```python
from build123d import *

# Parameters (mm, degrees)
SKETCH1_W           = 28
SKETCH1_H           = 12
BOSS_EXTRUDE1_DEPTH = 5
SKETCH2_W           = 28
SKETCH2_H           = 6
BOSS_EXTRUDE2_DEPTH = 13.5
SKETCH3_R           = 1.75
CUT_EXTRUDE1_DEPTH  = 21.353132437


with BuildPart() as part:
    # Sketch1 → Boss-Extrude1 (new body)
    with BuildSketch(Plane.XY):
        Rectangle(SKETCH1_W, SKETCH1_H)
    extrude(amount=BOSS_EXTRUDE1_DEPTH)

    # Sketch2 → Boss-Extrude2 (add)
    with BuildSketch(Plane.XY.offset(5)):
        with Locations((0, -3)):
            Rectangle(SKETCH2_W, SKETCH2_H)
    extrude(amount=BOSS_EXTRUDE2_DEPTH)

    # Sketch3 → Cut-Extrude1 (cut, through all)
    with BuildSketch(Plane.XY.offset(5)):
        with Locations((-11, 3)):
            Circle(SKETCH3_R)
        with Locations(Location((11, 3, 0), (0, 0, 180))):
            Circle(SKETCH3_R)
    extrude(amount=-CUT_EXTRUDE1_DEPTH, mode=Mode.SUBTRACT)


solid = part.part
```
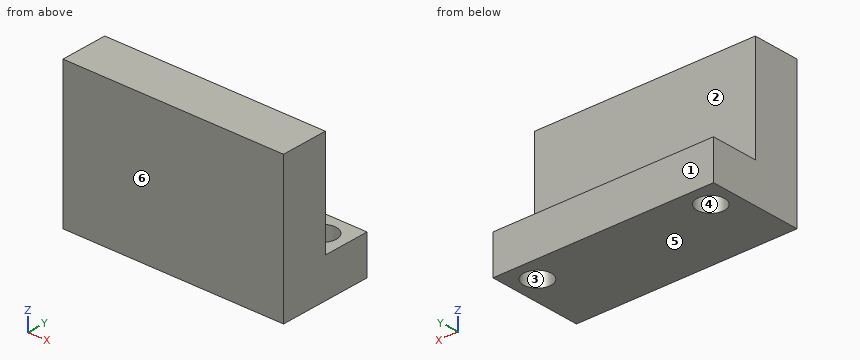
Check sheet for the modelled part. Datum: model origin and axes. Units: mm. Face numbers are marked on the shaded views. A direction names the side the tool comes from. Give positions to 0.01 mm unless a question says otherwise; leave off trailing zeros. Order: outer loops, then holes, each group sorted by start corner. A loop starts at its lowest first (then second) coordinate and runs counter-clockwise, first axis right, second up. Notation, with made-up numbers: M 30.25,18 L 89.25,18 A17 ccw 89.25,34 Z; hole C 71,19.5 d11. An arc over 180 degrees is marked long. Answer in a Markdown table with one row per item. Add a question column.
Q1. Sectioned sample at A-A, the plane x = 11. Record the boundary of the cut face in (y, z), and give its area (4 significant figures).
Q2. Release check for a two-part mould opening along Y. For the marked faces 3, 4, 5 and 6 record: released by +Y, released by -Y, zero draft, split by the parting line, or undercut.
Q3. Thickness scan on L1, parallel to Y at x = -11, z = 3.85; L2, parallel to Z at x = 0.5, y = 0.5; L3, parallel to Y at x = 3.5, z = 13.25. Record the ranges inside material, lowest first.
Q4. Sectioned sample at D-D, the plane x = -4. Record the boundary of the cut face in (y, z).
Q5. Sectioned sample at C-C, the plane z = 2. Record the boundary of the cut face in (x, y), and give its area (3 significant figures).
Q6. Access from +Z, -Z, +X, -X, +Y, -Y to the whole of each face (thin tool, end or side, straight path). Record for the marked faces 1 and 2.
Q7. Gauge pin test, flat ends, axial feed: pin 1 Ø1 at (x, y) = (10.5, -3) entering from -Z; pin 2 Ø1.5 at (x, z) = (6.5, 12) entering from +Y; pin 3 Ø3 at (x, y) = (-11, 3) entering from -Z; pin 4 Ø1.8 at (x, y) = (-6.5, 2) entering from +Z. Record the tip position at first contact, or that the pin passes through.
Q8. Sectioned sample at B-B, the plane y = 3. Record the boundary of the cut face in (x, z), and give its area (3 significant figures).
Verdict:
| question | item | result |
|---|---|---|
| 1 | outline | M -6,0 L 1.25,0 L 1.25,5 L 0,5 L 0,18.5 L -6,18.5 Z; M 4.75,0 L 6,0 L 6,5 L 4.75,5 Z |
| 1 | area | 123.5 mm² |
| 2 | face 3 | undercut |
| 2 | face 4 | undercut |
| 2 | face 5 | zero draft |
| 2 | face 6 | released by -Y |
| 3 | L1 | -6 to 1.25, 4.75 to 6 |
| 3 | L2 | 0 to 5 |
| 3 | L3 | -6 to 0 |
| 4 | outline | M -6,0 L 6,0 L 6,5 L 0,5 L 0,18.5 L -6,18.5 Z |
| 5 | outline | M -14,-6 L 14,-6 L 14,6 L -14,6 Z; hole C -11,3 d3.5; hole C 11,3 d3.5 |
| 5 | area | 317 mm² |
| 6 | face 1 | +Z, -Z, +X, -X, +Y |
| 6 | face 2 | +Z, +X, -X, +Y |
| 7 | pin 1 | z = 0 |
| 7 | pin 2 | y = 0 |
| 7 | pin 3 | through |
| 7 | pin 4 | z = 5 |
| 8 | outline | M -14,0 L -12.75,0 L -12.75,5 L -14,5 Z; M -9.25,0 L 9.25,0 L 9.25,5 L -9.25,5 Z; M 12.75,0 L 14,0 L 14,5 L 12.75,5 Z |
| 8 | area | 105 mm² |
